Design review of the part built by this model. Coordinates are the model's own, in mm. Coordinates: 2 decimals unless noted, no trailing zeros. Loops run counter-clockwise (first coordinate to the right, second up) from the corner with the lowest first, then second, coordinate; pieces in that order, holes last. Notation, with made-up numbers: (67.25, 62.5) -> (95.25, 62.5) arc R17 ccw to (95.25, 89.5) -> close; hole circle Ø9 at (-4, 56.25). An arc over 180 degrees is marked (long way). Answer in a Markdown table with one row per item.
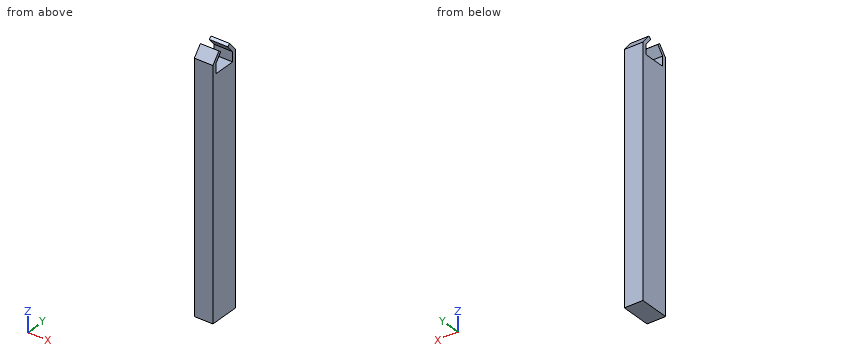
```python
from build123d import *

# Parameters (mm, degrees)
SKETCH1_W           = 19
SKETCH1_H           = 31
BOSS_EXTRUDE1_DEPTH = 240
BOSS_EXTRUDE2_DEPTH = 19


with BuildPart() as part:
    # Sketch1 → Boss-Extrude1 (new body)
    with BuildSketch(Plane.XY):
        Rectangle(SKETCH1_W, SKETCH1_H)
    extrude(amount=BOSS_EXTRUDE1_DEPTH)

    # Sketch2 → Boss-Extrude2 (add)
    with BuildSketch(Plane.ZY.offset(9.5)):
        Polygon((240, 15.5), (250, 15.5), (260, 7.226546943), (257.968239385, 4.770788022), (250, 11.363273472), (240, 11.363273472), align=None)
        Polygon((240, -15.5), (240, -11.363273472), (250, -11.363273472), (257.968239385, -4.770788022), (260, -7.226546943), (250, -15.5), align=None)
    extrude(amount=-BOSS_EXTRUDE2_DEPTH)


solid = part.part
```
(1) To check wall thickness, follow probe 1 along Y at (x, z) = (4.75, 242.5); probe 2 along Z at (x, y) = (0, -2); probe 3 along Z at (x, y) = (3.75, -5.5). State the ranges of each line that lie inside material, in increasing order.
Evaluation:
| item | result |
|---|---|
| probe 1 | y = -15.5 to -11.36, 11.36 to 15.5 |
| probe 2 | z = 0 to 240 |
| probe 3 | z = 0 to 240, 257.09 to 258.57 |
(2) Take a section at B-B on y = -2. Give the boundary of the cut face in (x, z).
Evaluation:
| item | result |
|---|---|
| outline | (-9.5, 0) -> (9.5, 0) -> (9.5, 240) -> (-9.5, 240) -> close |
(3) For pin 1 (9.5 mm diameter, centred on x = 0.5, y = -1.5, fed in from +Z); pin 2 (1 mm diameter, centred on x = 0.5, y = 6, fed in from -Z); pin 3 (1 mm diameter, centred on x = -3.5, y = 4.5, fed in from +Z), all flat-tipped, find the tip position at first contact; note any pin that passes through.
Evaluation:
| item | result |
|---|---|
| pin 1 | stops at z = 259.19 |
| pin 2 | stops at z = 0 |
| pin 3 | stops at z = 258.16 |
(4) Take a section at A-A on x = 5.75. Give the boundary of the cut face in (y, z), and give its area (3 significant figures).
Evaluation:
| item | result |
|---|---|
| outline | (-15.5, 0) -> (15.5, 0) -> (15.5, 250) -> (7.23, 260) -> (4.77, 257.97) -> (11.36, 250) -> (11.36, 240) -> (-11.36, 240) -> (-11.36, 250) -> (-4.77, 257.97) -> (-7.23, 260) -> (-15.5, 250) -> close |
| area | 7,600 mm² |
